Geometry: see drawing. Coordinates: mm, zero at the bounding-box minimum. A direction names the side the tool comes from. Give positions to 0.01 mm unless a question says otherwise; leave off trailing zeros. Write each loop counter-clockwise with the first axis right and the second up, starting at its lowest first coordinate (ties: lowest second). Pieces come first, ordered by that corner, then holes. Notation, with made-up numbers: M 78.5,-38 L 88.5,-38 A24 ccw 88.5,-12 Z; hole C 14.25,64 d4. An arc over 180 degrees is marked long. Use a Markdown table: item, result. Add a question column.
(1) Reachability of the marked faces 1 and 2 from +Z, -Z, +X, -X, +Y, -Y: full face, straight path, thin tool, end or side. Return the list, or none.
(2) Cut plane A-A (y = 25.5). Output: boundary loops of the cut face in (x, z).
(3) Cut plane C-C (x = 0.75). Output: boundary loops of the cut face in (y, z).
(4) Material intervals for L1, parallel to X at y = 4, z = 2.5 (1 decimal); L2, parallel to Z at x = 4, y = 11.5; L3, parallel to Y at x = 6, z = 1.5, sorted ascending.
(5) Cut plane B-B (z = 5.5). Output: boundary loops of the cut face in (x, y) (1 decimal).
(6) Pin query (flat end, axial travel): pin 1 Ø2 at (y, z) = (11.5, 1.5) entering from -X (1 decimal); pin 2 Ø1 at (x, z) = (4, 5) entering from -Y; pin 3 Ø3 at (x, y) = (2, 20) entering from -Z; pin 4 Ø2 at (x, y) = (4, 22.5) entering from +Z. Return the tip coordinate at first contact, or that it passes through.
(7) Cut plane D-D (y = 6.5). Output: boundary loops of the cut face in (x, z), plus the area to 3 significant figures.
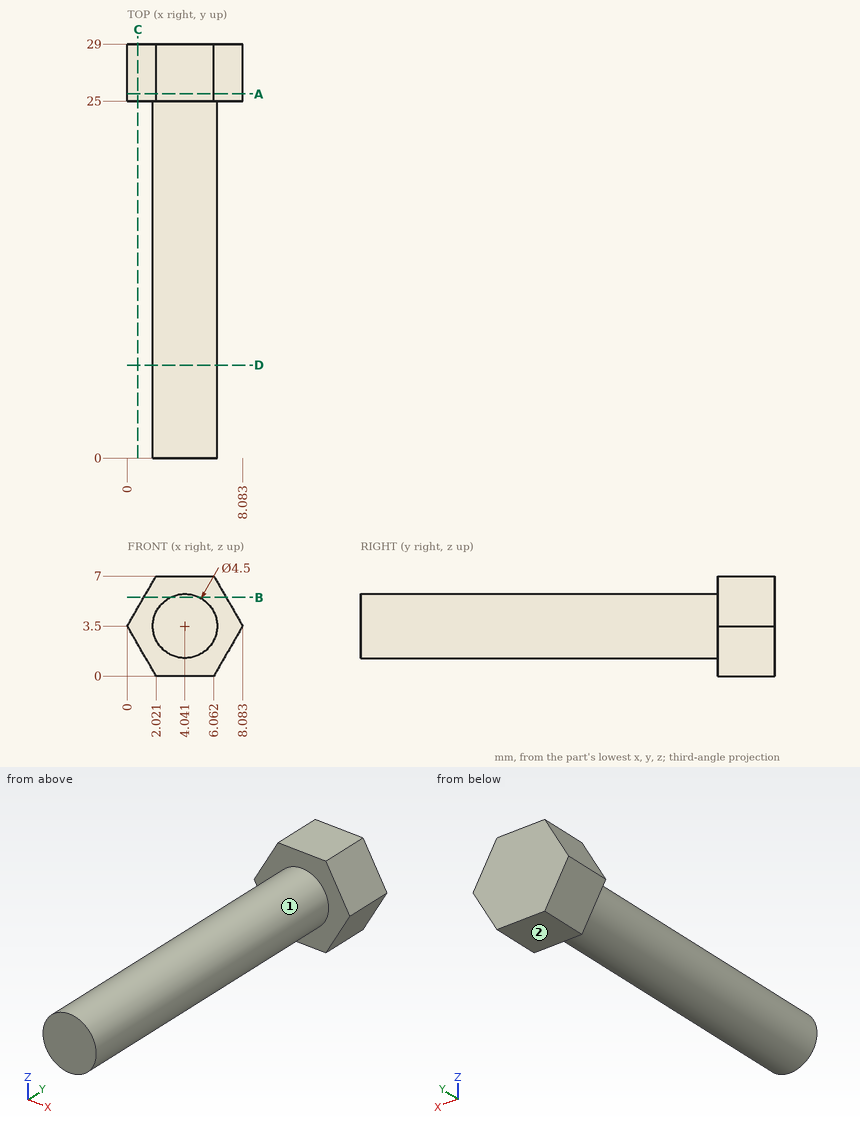
Answer list:
| question | item | result |
|---|---|---|
| 1 | face 1 | -Y |
| 1 | face 2 | -Z, +X, -X, +Y, -Y |
| 2 | outline | M 0,3.5 L 2.02,0 L 6.06,0 L 8.08,3.5 L 6.06,7 L 2.02,7 Z |
| 3 | outline | M 25,2.2 L 29,2.2 L 29,4.8 L 25,4.8 Z |
| 4 | L1 | 2 to 6.1 |
| 4 | L2 | 1.25 to 5.75 |
| 4 | L3 | 25 to 29 |
| 5 | outline | M 1.2,25 L 3,25 L 3,0 L 5.1,0 L 5.1,25 L 6.9,25 L 6.9,29 L 1.2,29 Z |
| 6 | pin 1 | x = 2 |
| 6 | pin 2 | y = 0 |
| 6 | pin 3 | z = 1.32 |
| 6 | pin 4 | z = 5.75 |
| 7 | outline | C 4.04,3.5 d4.5 |
| 7 | area | 15.9 mm² |
